Work out the finished part from the listing and answer in its coordinate system (mm). A direction names the side the tool comes from. Give positions to 0.01 mm unless a question says otherwise; leave off trailing zeros. Order: outer loops, then holes, each group sorted by start corner. A loop starts at its lowest first (then second) coordinate and runs counter-clockwise, first axis right, second up. Notation, with made-up numbers: (19.25, 52) - (46.25, 52) arc R31 ccw to (46.25, 91) - close; hole circle Ø5 at (59.25, 73). An arc over 180 degrees is marked (long way). Write each question's results on one line, items separated by ' | '.
from build123d import *

# Parameters (mm, degrees)
F0_W      = 39
F0_H      = 48
F1_DEPTH  = 5
F2_W      = 10
F2_H      = 32
F3_DEPTH  = 5.001
F4_W      = 39
F4_H      = 8
F5_DEPTH  = 30
F7_DEPTH  = 39
F8_R      = 4
F9_DEPTH  = 39.001
F10_R     = 1
F11_SIZE  = 4
F12_W     = 39
F12_H     = 8
F13_DEPTH = 8
F15_DEPTH = 35.001
F16_R     = 1
F17_R     = 5
F18_R     = 0.6
F19_W     = 7.55
F19_H     = 2.5
F20_DEPTH = 10
F21_SIZE2 = 9.99999
F21_SIZE  = 2.49999
F22_SIZE2 = 2.49999
F22_SIZE  = 9.99999


# Not quite as in the source:
# - a fillet or chamfer is up to 0.001 mm smaller than in the source, because OpenCascade refuses the exact size


with BuildPart() as f1:
    # F0 (on Front) → F1 (new body)
    with BuildSketch(Plane.XZ):
        with Locations((-5.5, 0)):
            Rectangle(F0_W, F0_H)
    extrude(amount=F1_DEPTH)

    # F2 (on face) → F3 (cut, through all)
    with BuildSketch(Plane.XZ.offset(5)):
        with Locations((-20, 0)):
            Rectangle(F2_W, F2_H)
        with Locations((9, 0)):
            Rectangle(F2_W, F2_H)
    extrude(amount=-F3_DEPTH, mode=Mode.SUBTRACT)

    # F4 (on face) → F5 (join)
    with BuildSketch(Plane(origin=(0, 0, 0), x_dir=(-1, 0, 0), z_dir=(0, 1, 0))):
        with Locations((5.5, 20)):
            Rectangle(F4_W, F4_H)
    extrude(amount=F5_DEPTH)

    # F6 (on face) → F7 (join, through all)
    with BuildSketch(Plane.YZ.offset(14)):
        Polygon((30, 16), (10, 16), (30, 15.2), align=None)
    extrude(amount=-F7_DEPTH)

    # F8 (on face) → F9 (cut, through all)
    with BuildSketch(Plane.YZ.offset(14)):
        with Locations((-5, 24)):
            Circle(F8_R)
    extrude(amount=-F9_DEPTH, mode=Mode.SUBTRACT)

    # F10
    f10_edges = [f1.edges().sort_by_distance(p)[0] for p in [
        (-5.5, -1, 24),
        (-5.5, -5, 20),
    ]]
    fillet(f10_edges, radius=F10_R)

    # F11
    f11_edges = [f1.edges().sort_by_distance(p)[0] for p in [
        (-5.5, 30, 24),
    ]]
    chamfer(f11_edges, length=F11_SIZE)

    # F12 (on face) → F13 (join)
    with BuildSketch(Plane(origin=(0, 0, 0), x_dir=(-1, 0, 0), z_dir=(0, 1, 0))):
        with Locations((5.5, -20)):
            Rectangle(F12_W, F12_H)
    extrude(amount=F13_DEPTH)

    # F14 (on face) → F15 (cut, through all)
    with BuildSketch(Plane.XZ.offset(5)):
        with BuildLine():
            Line((-3.55, -14.05), (-3.55, 13))
            ThreePointArc((-3.55, 13), (-5.5, 14.95), (-7.45, 13))
            Line((-7.45, 13), (-7.45, -14.05))
            ThreePointArc((-7.45, -14.05), (-5.5, -16), (-3.55, -14.05))
        make_face()
    extrude(amount=-F15_DEPTH, mode=Mode.SUBTRACT)

    # F16
    f16_edges = [f1.edges().sort_by_distance(p)[0] for p in [
        (-5.5, -4.2, 20.080816),
        (-5.5, -5, -24),
        (-25, -5, -20),
        (14, -5, -20),
        (14, -5, 17.55051),
        (-25, -5, 17.55051),
        (-25, 12.94949, 24),
        (14, 12.94949, 24),
        (14, 1.5, -24),
        (-25, 1.5, -24),
        (-5.5, 8, -16),
        (-5.5, 8, -24),
        (14, 8, -20),
        (-25, 8, -20),
        (-25, 1.5, -16),
        (14, 1.5, -16),
    ]]
    fillet(f16_edges, radius=F16_R)

    # F17
    f17_edges = [f1.edges().sort_by_distance(p)[0] for p in [
        (-15, -2.5, 16),
        (-15, -2.5, -16),
        (4, -2.5, 16),
        (4, -2.5, -16),
    ]]
    fillet(f17_edges, radius=F17_R)

    # F18
    f18_edges = [f1.edges().sort_by_distance(p)[0] for p in [
        (-5.5, 30, 15.2),
    ]]
    fillet(f18_edges, radius=F18_R)

    # F19 (on face) → F20 (join)
    with BuildSketch(Plane(origin=(0, 0, 0), x_dir=(-1, 0, 0), z_dir=(0, 1, 0))):
        with Locations((-0.225, 14.75)):
            Rectangle(F19_W, F19_H)
        with Locations((11.225, 14.75)):
            Rectangle(F19_W, F19_H)
    extrude(amount=F20_DEPTH)

    # F21 (size 2.5 and 10 in the source; OpenCascade refuses exactly that, so slightly less here)
    f21_edges = [f1.edges().sort_by_distance(p)[0] for p in [
        (0.225, 10, 13.5),
    ]]
    f21_side = f1.faces().sort_by_distance((0.225, 10, 14.75))[0]
    chamfer(f21_edges, length=F21_SIZE, length2=F21_SIZE2, reference=f21_side)

    # F22 (size 10 and 2.5 in the source; OpenCascade refuses exactly that, so slightly less here)
    f22_edges = [f1.edges().sort_by_distance(p)[0] for p in [
        (-11.225, 10, 13.5),
    ]]
    f22_side = f1.faces().sort_by_distance((-11.225, 5, 13.5))[0]
    chamfer(f22_edges, length=F22_SIZE, length2=F22_SIZE2, reference=f22_side)


solid = f1.part
1. Given P1, Ø3, axis at x = -7.5, z = -13, coming from the +Y side; P2, Ø1.5, axis at y = -3, z = 6, coming from the +X side; P3, Ø4, axis at y = -3.5, z = -0.5, coming from the -X side, each flat-ended and moving along its own axis, determine where each tip first touches the part or whether it passes through.
Answer list:
P1: y = 0 | P2: x = 4 | P3: x = -15
2. A cutting plane is placed at D-D, the plane x = -16.5. Write down the section's boundary in (y, z).
Answer list:
outline: (-5, -23) arc R1 ccw to (-4, -24) - (7, -24) arc R1 ccw to (8, -23) - (8, -17) arc R1 ccw to (7, -16) - (0, -16) - (0, -14.57) - (-5, -14.57) - close; (-5, 14.57) - (0, 14.57) - (0, 16) - (10, 16) - (29.38, 15.22) arc R0.6 ccw to (30, 15.82) - (30, 20) - (26, 24) - (-0.1, 24) arc R1 ccw to (-1.08, 23.2) arc R4 cw to (-4.2, 20.08) arc R1 ccw to (-5, 19.1) - close
3. Straight lines are drawn through the part: line 1 (Y direction, x = -11.5, z = -14); line 2 (Y direction, x = -15, z = -18); line 3 (Z direction, x = -21.5, y = -2.5). For each, find the intervals that lie inside material, in ascending order. Write a range as [from, to].
Answer list:
line 1: [-5, 0] | line 2: [-5, 8] | line 3: [-24, -16], [16, 20.88]
4. A tool of negligible diameter and unlimited length cuts with its end or side. For faces 4 (the face through (-17, -2, 15)), 5 (the face through (-15, 4, 15)), 6 (the face through (-5.5, -2.5, -16)), from which of +Z, -Z, +X, -X, +Y, -Y can it reach the whole face along a straight path? Write none if from no direction.
Answer list:
face 4: -X, -Y | face 5: -X | face 6: +Y, -Y
5. Determine the mould class of faces 1 (the face through (-5.23, 19.55, 15.62)), 2 (the face through (14, 1, -20)), 3 (the face through (-17, -2, -15)) for opening direction Z: +Z half, -Z half, draft (parallel to the pull), parting line (faces both ways), or undercut.
Answer list:
face 1: -Z half | face 2: draft | face 3: undercut
6. A cutting plane is placed at B-B, the plane y = 1. Write down the section's boundary in (x, z), then the cut area to 3 significant figures.
Answer list:
outline: (-25, -23) arc R1 ccw to (-24, -24) - (13, -24) arc R1 ccw to (14, -23) - (14, -17) arc R1 ccw to (13, -16) - (-24, -16) arc R1 ccw to (-25, -17) - close; (-25, 16) - (-15, 16) - (-15, 13.75) - (-7.45, 13.75) - (-7.45, 16) - (-3.55, 16) - (-3.55, 13.75) - (4, 13.75) - (4, 16) - (14, 16) - (14, 23) arc R1 ccw to (13, 24) - (-24, 24) arc R1 ccw to (-25, 23) - close | area: 657 mm^2
7. A cutting plane is placed at C-C, the plane z = -12. Write down the section's boundary in (x, y).
Answer list:
outline: (-15.1, -5) - (-7.45, -5) - (-7.45, 0) - (-15.1, 0) - close; (-3.55, -5) - (4.1, -5) - (4.1, 0) - (-3.55, 0) - close
